from build123d import *

# Parameters (mm, degrees)
SKETCH1_W           = 20
SKETCH1_H           = 20
BOSS_EXTRUDE1_DEPTH = 3
SKETCH2_W           = 10
SKETCH2_H           = 10
CUT_EXTRUDE1_DEPTH  = 1
FILLET1_R           = 1


with BuildPart() as part:
    # Sketch1 → Boss-Extrude1 (new body)
    with BuildSketch(Plane(origin=(0, 0, 0), x_dir=(1, 0, 0), z_dir=(0, 1, 0))):
        Rectangle(SKETCH1_W, SKETCH1_H)
    extrude(amount=BOSS_EXTRUDE1_DEPTH)

    # Sketch2 → Cut-Extrude1 (cut)
    with BuildSketch(Plane(origin=(0, 3, 0), x_dir=(1, 0, 0), z_dir=(0, 1, 0))):
        Rectangle(SKETCH2_W, SKETCH2_H)
    extrude(amount=-CUT_EXTRUDE1_DEPTH, mode=Mode.SUBTRACT)

    # Fillet1
    fillet1_edges = [part.edges().sort_by_distance(p)[0] for p in [
        (-5, 2.5, 5),
        (-5, 2.5, -5),
        (5, 2.5, -5),
        (5, 2.5, 5),
        (-10, 1.5, -10),
        (10, 1.5, -10),
        (10, 1.5, 10),
        (-10, 1.5, 10),
    ]]
    fillet(fillet1_edges, radius=FILLET1_R)


solid = part.part
The listing builds one solid part. Answer for the finished solid, in the listing's coordinates (mm). A direction names the side the tool comes from. Give positions to 0.01 mm unless a question says otherwise; leave off trailing zeros. Loops run counter-clockwise (first coordinate to the right, second up) from the corner with the lowest first, then second, coordinate; pieces in that order, holes last. Notation, with made-up numbers: (3.5, 15) - (24.5, 15) arc R22 ccw to (24.5, 34) - close; hole circle Ø1 at (69, 72). An arc over 180 degrees is marked (long way). Write each question's results on one line, items separated by ' | '.
1. Find section B-B, the plane x = 2.5. Write down the section's boundary in (y, z).
Resolved:
outline: (0, -10) - (3, -10) - (3, -5) - (2, -5) - (2, 5) - (3, 5) - (3, 10) - (0, 10) - close
2. Flat-ended cylindrical pins translate along their axes: P1, Ø8, axis at x = 2, z = -1, coming from the +Y side; P2, Ø5, axis at x = -0.5, z = 0, coming from the +Y side. Find the tip coordinate at first contact, or state that the pin passes through.
Resolved:
P1: stops at y = 3 | P2: stops at y = 2
3. Which of the six approach directions +Z, -Z, +X, -X, +Y, -Y give full straight-line access (tool end or side, diameter ignored) to faces 5 (the face through (-0.1, 2.5, 5)), 6 (the face through (0, 0, 0))?
Resolved:
face 5: +Y | face 6: +Z, -Z, +X, -X, -Y
4. Find section A-A, the plane z = 2. Write down the section's boundary in (x, y).
Resolved:
outline: (-10, 0) - (10, 0) - (10, 3) - (5, 3) - (5, 2) - (-5, 2) - (-5, 3) - (-10, 3) - close
5. Consider probe 1 along Z at (x, y) = (3.75, 2.5); probe 2 along Y at (x, z) = (0.5, -1.75). Determine where each line is inside the solid, lowest interval first. Write a range as from..to.
Resolved:
probe 1: z = -10..-5, 5..10 | probe 2: y = 0..2
6. Find section C-C, the plane y = 2.5. Write down the section's boundary in (x, z), then the cut area to 3 significant figures.
Resolved:
outline: (-10, -9) arc R1 ccw to (-9, -10) - (9, -10) arc R1 ccw to (10, -9) - (10, 9) arc R1 ccw to (9, 10) - (-9, 10) arc R1 ccw to (-10, 9) - close; hole (-5, -4) arc R1 ccw to (-4, -5) - (4, -5) arc R1 ccw to (5, -4) - (5, 4) arc R1 ccw to (4, 5) - (-4, 5) arc R1 ccw to (-5, 4) - close | area: 300 mm^2
7. For a pull along X with two mould halves and no side action, classify faces 1 (the face through (5, 2.5, 0.1)), 2 (the face through (0, 3, -7)), 3 (the face through (-4.699, 2.493, -4.715)), 4 (the face through (9.699, 1.521, 9.715)) as +X half, -X half, draft (parallel to the pull), parting line (faces both ways), or undercut.
Resolved:
face 1: undercut | face 2: draft | face 3: undercut | face 4: +X half
